Source: CAD feature listing. Evaluate the final solid. Frame: model axes, mm. Face numbers are marked on the shaded views. A direction names the side the tool comes from. Give positions to 0.01 mm unless a question says otherwise; leave off trailing zeros. Write each loop counter-clockwise with the first axis right and the second up, starting at its lowest first coordinate (ties: lowest second). Pieces come first, ordered by that corner, then holes. Notation, with made-up numbers: (82.25, 45) -> (110.25, 45) arc R19 cw to (110.25, 50) -> close; hole circle Ø7 at (55, 28.5). An arc over 180 degrees is marked (long way). Write item = value, one per line.
Autodesk Inventor part; units mm, degrees
ref_plane "YZ Plane" through (0, 0, 0) normal (1, 0, 0) x (0, 1, 0)
ref_plane "XZ Plane" through (0, 0, 0) normal (0, 1, 0) x (-1, 0, 0)
ref_plane "XY Plane" through (0, 0, 0) normal (0, 0, 1) x (1, 0, 0)
sketch "Sketch1" plane through (0, 0, 0) normal (0, 1, 0) x (-1, 0, 0)
  circle A0 centre (0, 0) radius 3.683
  dimension "d0" = 7.366
extrude "Extrusion1" add sketch "Sketch1" along normal blind 1.27
sketch "Sketch2" plane through (0, 1.27, 0) normal (0, 1, 0) x (1, 0, 0)
  circle A0 centre (0, 0) radius 1.5875
  dimension "d3" = 3.175
extrude "Extrusion2" add sketch "Sketch2" along normal blind 40.64
sketch "Sketch3" plane through (0, 41.91, 0) normal (0, 1, 0) x (1, 0, 0)
  line L0 (3.683, 3.683) -> (-3.683, 3.683)
  line L1 (-3.683, 3.683) -> (-3.683, -3.683)
  line L2 (-3.683, -3.683) -> (3.683, -3.683)
  line L3 (3.683, -3.683) -> (3.683, 3.683)
  line L4 (3.683, 3.683) -> (-3.683, -3.683) construction
  line L5 (-3.683, 3.683) -> (3.683, -3.683) construction
  point P0 (0, 0)
extrude "Extrusion3" add sketch "Sketch3" along normal blind 7.62
sketch "Sketch4" plane through (3.683, 41.91, 3.683) normal (1, 0, 0) x (0, 0, -1)
  circle A0 centre (3.556, 3.81) radius 3.175
  line L0 (7.366, 7.62) -> (0, 7.62)
  line L1 (7.366, 0) -> (7.366, 7.62)
  point P0 (3.683, -41.91)
  dimension "d8" = 3.81
  dimension "d9" = 3.81
  dimension "d10" = 6.35
extrude "Extrusion4" cut sketch "Sketch4" against normal blind 7.62
fillet "Fillet1" radius 3.556 4 edges at (0, 41.91, 3.683) (0, 49.53, 3.683) (0, 49.53, -3.683) (0, 41.91, -3.683)
properties part number "piston2"
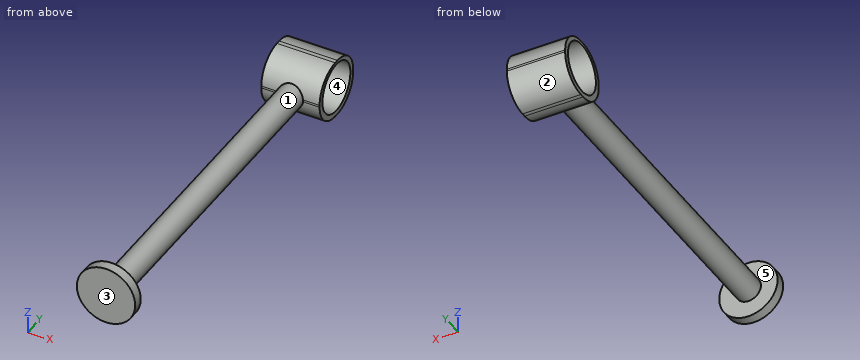
1) Draft query along Y for the marked faces 1, 2 and 3. Return one class per face: pulls with the +Y half, pulls with the -Y half, needs draft (parallel to the pull), parting line crosses it, or undercut.
Computed:
face_1 = undercut
face_2 = pulls with the +Y half
face_3 = pulls with the -Y half
2) Material intervals for L1, parallel to Y at x = 1.75, z = -1.25; L2, parallel to X at y = 13.5, z = 0; L3, parallel to Y at x = -2.25, z = 1.5, sorted ascending.
Computed:
L1 = 0 to 1.27, 42.09 to 42.86, 48.58 to 49.35
L2 = -1.59 to 1.59
L3 = 0 to 1.27, 42.19 to 42.86, 48.58 to 49.25
3) Cut plane B-B (x = -2.5). Return the cut outline in (y, z) (3 decimals).
Computed:
outline = (0, -2.705) -> (1.27, -2.705) -> (1.27, 2.705) -> (0, 2.705) -> close; (41.91, -0.127) arc R3.556 ccw to (45.466, -3.683) -> (45.974, -3.683) arc R3.556 ccw to (49.53, -0.127) -> (49.53, 0.127) arc R3.556 ccw to (45.974, 3.683) -> (45.466, 3.683) arc R3.556 ccw to (41.91, 0.127) -> close; hole circle Ø6.35 at (45.72, 0.127)
4) Access query for the marked faces 4 and 5. Directions: +Z, -Z, +X, -X, +Y, -Y. A direction counts if a zero-diameter tool reaches every point of the face in a straight line with its end or side. Return the directions, or none.
Computed:
face_4 = +X, -X
face_5 = none
5) Cut plane C-C (y = 43). Return the cut outline in (x, z), then the cut area to 3 significant figures.
Computed:
outline = (-3.68, -2.69) -> (3.68, -2.69) -> (3.68, -1.51) -> (-3.68, -1.51) -> close; (-3.68, 1.76) -> (3.68, 1.76) -> (3.68, 2.69) -> (-3.68, 2.69) -> close
area = 15.5 mm²
6) Contact query for flat-ended pins moving along their axis: pin 1 (4 mm diameter, centred on y = 36.5, z = 3, fed in from +X); pin 2 (2 mm diameter, centred on y = 26.5, z = 2, fed in from -X); pin 3 (2 mm diameter, centred on x = 1, z = 2.5, fed in from +Y). Output: stop coordinate, or through.
Computed:
pin_1 = 1.23
pin_2 = -1.23
pin_3 = 49.25
7) Cut plane D-D (y = 11). Return the cut outline in (x, z) (1 decimal), then the cut area to 3 significant figures.
Computed:
outline = circle Ø3.2 at (0, 0)
area = 7.92 mm²
